The drawing under review shows one solid part. Ordinate dimensions are in mm from its lowest x, y, z. A direction names the side the tool comes from. Give positions to 0.01 mm unless a question says otherwise; leave off trailing zeros. Loops run counter-clockwise (first coordinate to the right, second up) from the corner with the lowest first, then second, coordinate; pieces in that order, holes last. Notation, with made-up numbers: M 30,13 L 38,13 A21 ccw 38,47 Z; hole C 68,35 d7. An arc over 180 degrees is marked long. Write item = value, one per line. Start each with the question number.
1. We need section B-B on z = 42.5. Give the boundary of the cut face in (x, y) (1 decimal), then the cut area to 3 significant figures.
2. We need section D-D on y = 83. Give the boundary of the cut face in (x, z) (1 decimal).
3. Wall thickness on line 1 along X through (y, z) = (78, 54) (1 decimal); line 2 along Z through (x, y) = (35, 77.5) (1 decimal); line 3 along Y through (x, z) = (57.5, 41.5) (1 decimal): over which ranges is each line inside the solid? List them lowest first. Write a range as from..to.
4. For the marked faces 4, 5 and 6, list the 3-axis set-ups (+Z, -Z, +X, -X, +Y, -Y) from which the entire face can be reached by the end or side of a thin tool; tool diameter is ignored.
5. Draft analysis for pull direction Z (two halves, no side actions). For the marked faces 1, 2 and 3, state which applies: pulls with the +Z half, pulls with the -Z half, needs draft (parallel to the pull), parting line crosses it, or undercut.
6. We need section C-C on z = 16. Give the boundary of the cut face in (x, y) (1 decimal).
7. We need section A-A on x = 23. Give the boundary of the cut face in (y, z) (1 decimal).
8. For pin 1 (12 mm diameter, centred on x = 39, y = 42.5, fed in from -Z); pin 2 (6 mm diameter, centred on y = 71, z = 10, fed in from +X); pin 3 (12 mm diameter, centred on x = 50.5, y = 65, fed in from +Z), all flat-tipped, find the tip position at first contact; note any pin that passes through.
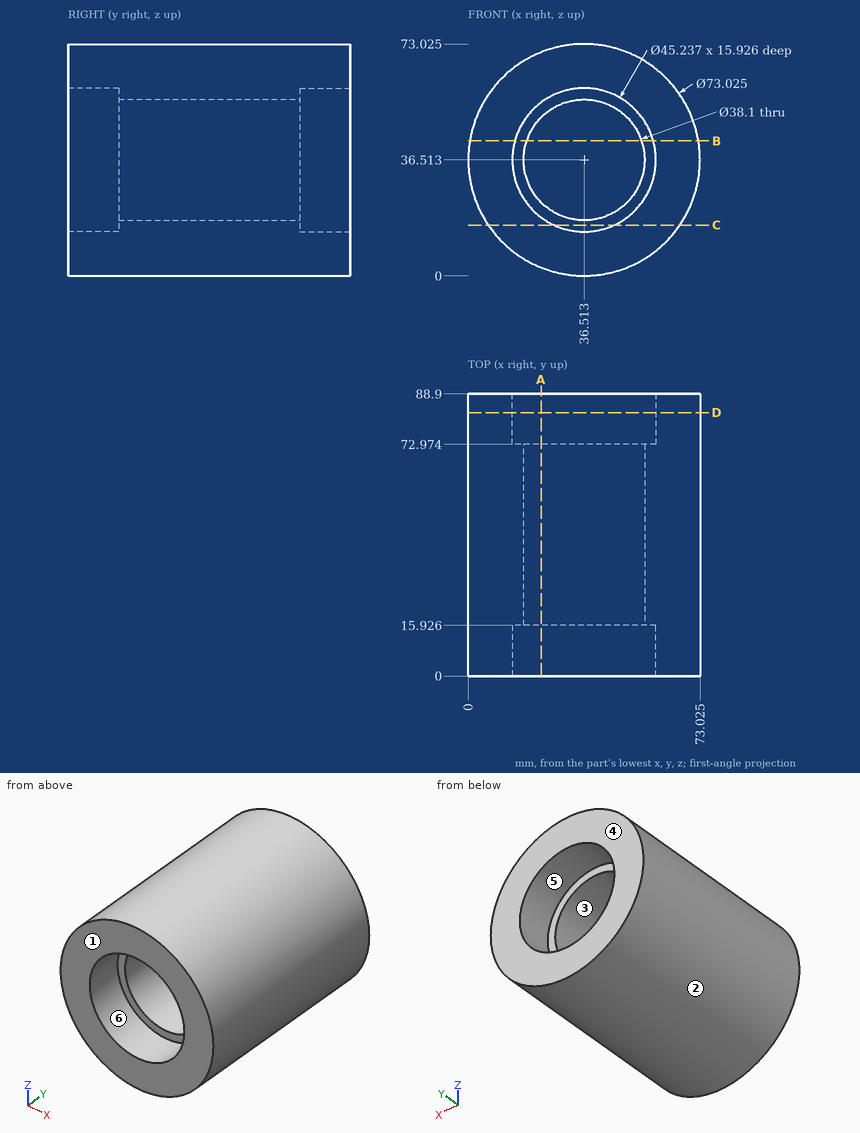
Final values:
q1.outline = M 0.5,0 L 14.7,0 L 14.7,15.9 L 18.4,15.9 L 18.4,73 L 14.7,73 L 14.7,88.9 L 0.5,88.9 Z; M 54.6,15.9 L 58.3,15.9 L 58.3,0 L 72.5,0 L 72.5,88.9 L 58.3,88.9 L 58.3,73 L 54.6,73 Z
q1.area = 2,950 mm²
q2.outline = C 36.5,36.5 d73; hole C 36.5,36.5 d45.2
q3.line_1 = 4.5..22.2, 50.9..68.6
q3.line_2 = 0..13.9, 59.1..73
q3.line_3 = 15.9..73
q4.face_4 = +Z, -Z, +X, -X, +Y
q4.face_5 = +Y
q4.face_6 = -Y
q5.face_1 = needs draft
q5.face_2 = parting line crosses it
q5.face_3 = undercut
q6.outline = M 6.3,0 L 27,0 L 27,15.9 L 46,15.9 L 46,0 L 66.7,0 L 66.7,88.9 L 46,88.9 L 46,73 L 27,73 L 27,88.9 L 6.3,88.9 Z
q7.outline = M 0,2.6 L 88.9,2.6 L 88.9,18.4 L 73,18.4 L 73,23.1 L 15.9,23.1 L 15.9,18.4 L 0,18.4 Z; M 0,54.7 L 15.9,54.7 L 15.9,49.9 L 73,49.9 L 73,54.7 L 88.9,54.7 L 88.9,70.4 L 0,70.4 Z
q8.pin_1 = 0
q8.pin_2 = 64.45
q8.pin_3 = 72.14
